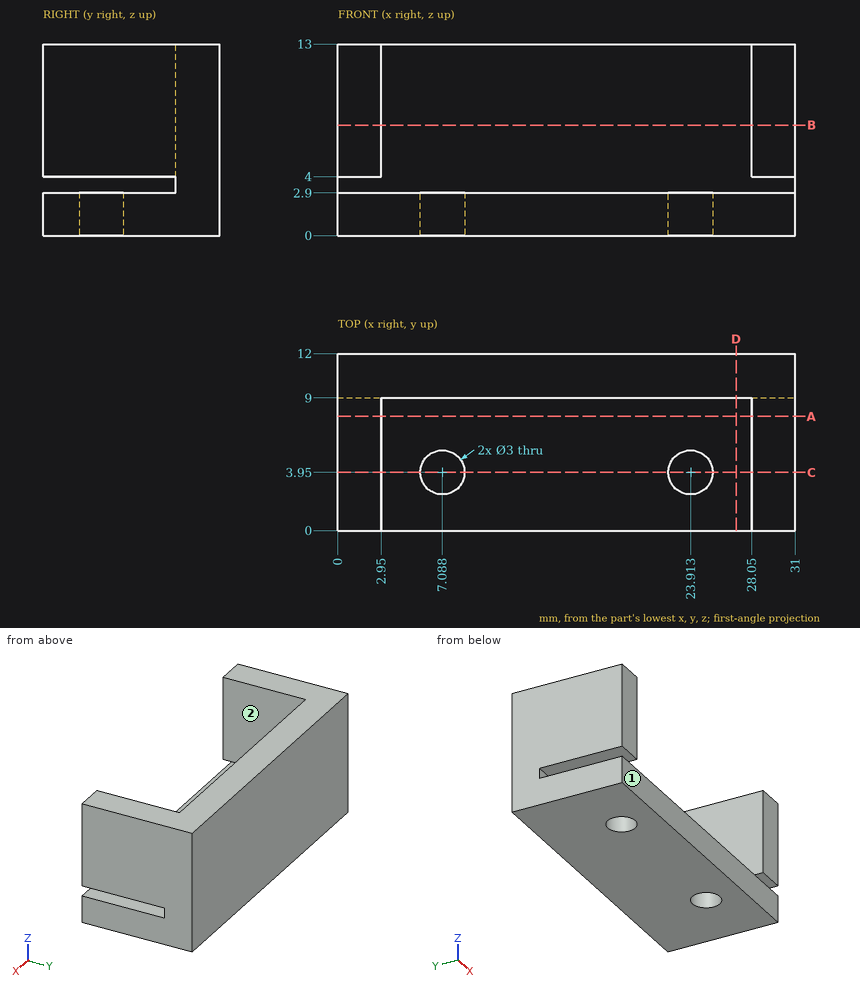
Part print with two shaded views. Sizes in mm from the minimum x, y, z corner. A direction names the side the tool comes from. Coordinates: 2 decimals unless noted, no trailing zeros. Write each loop counter-clockwise with the first axis right and the second up, starting at its lowest first coordinate (ties: lowest second). Pieces come first, ordered by that corner, then holes. Notation, with made-up numbers: M -4,-19.75 L 34,-19.75 A20 ccw 34,-14.75 Z; hole C -35.75,-4.5 d2. An arc over 180 degrees is marked long. Return JSON: item names as keys, results as strings.
Item 1: Which spindle directions (+Z, -Z, +X, -X, +Y, -Y) get a long thin tool onto all of the face, cutting with end or side? Do the marked faces 1 and 2. Say none if no direction does.
Findings below:
{"face 1": "+Z, -Z, +X, -X, -Y", "face 2": "+Z, -Y"}
Item 2: Slice it at D-D, the plane x = 27. Write the cut outline in (y, z).
Findings below:
{"outline": "M 0,0 L 12,0 L 12,13 L 9,13 L 9,2.9 L 0,2.9 Z"}
Item 3: Slice it at A-A, the plane y = 7.75. Write the cut outline in (x, z), and give its area (3 significant figures).
Findings below:
{"outline": "M 0,0 L 31,0 L 31,2.9 L 0,2.9 Z; M 0,4 L 2.95,4 L 2.95,13 L 0,13 Z; M 28.05,4 L 31,4 L 31,13 L 28.05,13 Z", "area": "143 mm2"}
Item 4: Drop flat-ended pins along their axis: pin 1 Ø2 at (x, z) = (26, 11) entering from -Y; pin 2 Ø4 at (x, y) = (7.09, 3.95) entering from +Z. Give the stop position or say it passes through.
Findings below:
{"pin 1": "stops at y = 9", "pin 2": "stops at z = 2.9"}
Item 5: Slice it at B-B, the plane z = 7.5. Write the cut outline in (x, y), and give its area (3 significant figures).
Findings below:
{"outline": "M 0,0 L 2.95,0 L 2.95,9 L 28.05,9 L 28.05,0 L 31,0 L 31,12 L 0,12 Z", "area": "146 mm2"}
Item 6: Slice it at C-C, the plane y = 3.95. Write the cut outline in (x, z).
Findings below:
{"outline": "M 0,0 L 5.59,0 L 5.59,2.9 L 0,2.9 Z; M 0,4 L 2.95,4 L 2.95,13 L 0,13 Z; M 8.59,0 L 22.41,0 L 22.41,2.9 L 8.59,2.9 Z; M 25.41,0 L 31,0 L 31,2.9 L 25.41,2.9 Z; M 28.05,4 L 31,4 L 31,13 L 28.05,13 Z"}
Item 7: Probe line 1 (X direction, y = 4.75, z = 8.5); line 2 (Z direction, x = 29.5, y = 5.5); line 3 (Z direction, x = 23, y = 5.75). List the from-to ranges inside material, lowest first. Write a range as from..to.
Findings below:
{"line 1": "x = 0..2.95, 28.05..31", "line 2": "z = 0..2.9, 4..13", "line 3": "z = 0..2.9"}
